Design review of the part built by this model. Coordinates are the model's own, in mm. Coordinates: 2 decimals unless noted, no trailing zeros. Loops run counter-clockwise (first coordinate to the right, second up) from the corner with the lowest first, then second, coordinate; pieces in that order, holes last. Notation, with made-up numbers: (22, 34) -> (80, 34) arc R16 cw to (80, 58) -> close; hole circle Ø3 at (48, 83). An arc over 180 degrees is marked (long way). Use a Markdown table: item, result. Add a question column.
Q1. Take a section at B-B on z = -4. Write out the cut boundary in (x, y).
Q2. Clearance check with flat-ended pins moving along their axes: pin 1 Ø1.5 at (y, z) = (-41.5, 1.5) entering from -X; pin 2 Ø3 at (y, z) = (14.5, 4.5) entering from -X; pin 3 Ø1.1 at (x, z) = (0, -1.5) entering from +Y. State where each tip first meets the part, or that it passes through.
Q3. For probe 1 along Z at (x, y) = (1, -110); probe 2 along Y at (x, z) = (0.5, -0.25); probe 3 along X at (y, z) = (-85, 0.25), list the stretches that pass through material, from the lowest coordinate up.
Q4. Take a section at A-A on y = -53. Write out the cut boundary in (x, z).
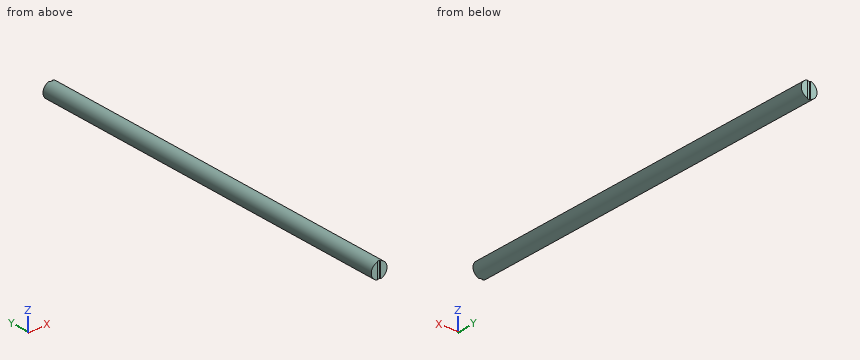
from build123d import *

# Parameters (mm, degrees)
F0_R     = 6.35
F1_DEPTH = 155.321
F2_W     = 2.286
F2_H     = 12.7
F3_DEPTH = 0.762
F4_W     = 2.286
F4_H     = 12.7
F5_DEPTH = 0.762


with BuildPart() as f1:
    # F0 (on Front) → F1 (new body, symmetric)
    with BuildSketch(Plane.XZ):
        Circle(F0_R)
    extrude(amount=F1_DEPTH, both=True)

    # F2 (on face) → F3 (cut)
    with BuildSketch(Plane.XZ.offset(155.321)):
        Rectangle(F2_W, F2_H)
    extrude(amount=-F3_DEPTH, mode=Mode.SUBTRACT)

    # F4 (on face) → F5 (cut)
    with BuildSketch(Plane(origin=(0, 155.321, 0), x_dir=(-1, 0, 0), z_dir=(0, 1, 0))):
        Rectangle(F4_W, F4_H)
    extrude(amount=-F5_DEPTH, mode=Mode.SUBTRACT)


solid = f1.part
Answer list:
| question | item | result |
|---|---|---|
| 1 | outline | (-4.93, -155.32) -> (-1.14, -155.32) -> (-1.14, -154.56) -> (1.14, -154.56) -> (1.14, -155.32) -> (4.93, -155.32) -> (4.93, 155.32) -> (1.14, 155.32) -> (1.14, 154.56) -> (-1.14, 154.56) -> (-1.14, 155.32) -> (-4.93, 155.32) -> close |
| 2 | pin 1 | x = -6.31 |
| 2 | pin 2 | x = -5.6 |
| 2 | pin 3 | y = 154.56 |
| 3 | probe 1 | -6.27 to 6.27 |
| 3 | probe 2 | -154.56 to 154.56 |
| 3 | probe 3 | -6.35 to 6.35 |
| 4 | outline | circle Ø12.7 at (0, 0) |
